```python
from build123d import *

# Parameters (mm, degrees)
BOSS_EXTRUDE1_DEPTH = 27
SHELL3_T            = -2
CUT_EXTRUDE1_DEPTH  = 2


with BuildPart() as part:
    # Sketch2 → Boss-Extrude1 (new body)
    with BuildSketch(Plane(origin=(0, 0, 0), x_dir=(1, 0, 0), z_dir=(0, 1, 0))):
        with BuildLine():
            Line((-18.993396104, 10.600093214), (-15.993396104, 10.600093214))
            ThreePointArc((-15.993396104, 10.600093214), (-12.085516583, 10.0001005), (-15.993393867, 9.400093214))
            Line((-15.993393867, 9.400093214), (-18.993393867, 9.400093214))
            ThreePointArc((-18.993393867, 9.400093214), (-19.274030957, 4.676202489), (-20, 0))
            Line((-20, 0), (0, 0))
            Line((0, 0), (0, 20))
            Line((0, 20), (-20, 20))
            ThreePointArc((-20, 20), (-19.274040883, 15.323890203), (-18.993396104, 10.600093214))
        make_face()
    extrude(amount=BOSS_EXTRUDE1_DEPTH)

    # Shell3
    shell3_openings = [part.faces().sort_by_distance(p)[0] for p in [
        (-19.274030957, 13.5, -4.676202489),
        (-17.493393867, 13.5, -9.400093214),
        (-12.085516583, 13.5, -10.0001005),
        (-17.493396104, 13.5, -10.600093214),
        (-19.274040883, 13.5, -15.323890203),
    ]]
    offset(amount=SHELL3_T, openings=shell3_openings, kind=Kind.INTERSECTION)

    # Sketch3 → Cut-Extrude1 (cut)
    with BuildSketch(Plane(origin=(0, 0, 0), x_dir=(0, 0, -1), z_dir=(1, 0, 0))):
        with BuildLine():
            ThreePointArc((12, 13.5), (10.89974713, 15.286184509), (8.809544899, 15.107114387))
            Line((8.809544899, 15.107114387), (11.190455101, 11.892885613))
            ThreePointArc((11.190455101, 11.892885613), (11.786184509, 12.60025287), (12, 13.5))
        make_face()
        with BuildLine():
            Line((11.190455101, 11.892885613), (8.809544899, 15.107114387))
            ThreePointArc((8.809544899, 15.107114387), (8.392885613, 12.309544899), (11.190455101, 11.892885613))
        make_face()
    extrude(amount=-CUT_EXTRUDE1_DEPTH, mode=Mode.SUBTRACT)


solid = part.part
```
Design review of the part built by this model. Coordinates are the model's own, in mm. A direction names the side the tool comes from. Coordinates: 2 decimals unless noted, no trailing zeros. Order: outer loops, then holes, each group sorted by start corner. A loop starts at its lowest first (then second) coordinate and runs counter-clockwise, first axis right, second up. Notation, with made-up numbers: (3.25, -20.75) - (25.25, -20.75) arc R21 cw to (25.25, -2.75) - close; hole circle Ø2 at (25, 68). An arc over 180 degrees is marked (long way). Answer in a Markdown table with one row per item.
(1) Clearance check with flat-ended pins moving along their axes: pin 1 (12 mm diameter, centred on y = 19, z = -13.5, fed in from -X); pin 2 (3.5 mm diameter, centred on x = -14.09, z = -10, fed in from -Y); pin 3 (4 mm diameter, centred on y = 13.5, z = -9.5, fed in from -X). State where each tip first meets the part, or that it passes through.
Checked values:
| item | result |
|---|---|
| pin 1 | x = -19.9 |
| pin 2 | through |
| pin 3 | x = -2 |
(2) Consider section B-B on x = -18. State the section outline as (y, z) points, plus the area to 3 significant figures.
Checked values:
| item | result |
|---|---|
| outline | (0, -20) - (27, -20) - (27, -10.6) - (25, -10.6) - (25, -18) - (2, -18) - (2, -10.6) - (0, -10.6) - close; (0, -9.4) - (2, -9.4) - (2, -2) - (25, -2) - (25, -9.4) - (27, -9.4) - (27, 0) - (0, 0) - close |
| area | 167 mm^2 |
(3) Wall thickness on line 1 along Y through (x, z) = (-6, -12); line 2 along Z through (x, y) = (-18.75, 8.5); line 3 along X through (y, z) = (21.75, -2.75): over which ranges is each line inside the solid? List them lowest first. Write a range as from..to.
Checked values:
| item | result |
|---|---|
| line 1 | 0..2, 25..27 |
| line 2 | -20..-18, -2..0 |
| line 3 | -2..0 |
(4) For faces 5 (the flat face through (-17, 1, -9.4)), 6 (the flat face through (-11, 13, -18)), 7 (the flat face through (-10, 27, -10)), list the 3-axis set-ups (+Z, -Z, +X, -X, +Y, -Y) from which the entire face can be reached by the end or side of a thin tool; tool diameter is ignored.
Checked values:
| item | result |
|---|---|
| face 5 | -X, +Y, -Y |
| face 6 | -X |
| face 7 | +Z, -Z, +X, -X, +Y |
(5) Consider section C-C on x = -9.25. State the section outline as (y, z) points.
Checked values:
| item | result |
|---|---|
| outline | (0, -20) - (27, -20) - (27, 0) - (0, 0) - close; hole (2, -18) - (25, -18) - (25, -2) - (2, -2) - close |
(6) The part is to be moulded in two halves that separate along Y. For faces 1 (the flat face through (-18, 26, -10.6)), 2 (the flat face through (-10, 0, -10)), 3 (the flat face through (-11, 25, -10)), 4 (the flat face through (-2, 16, -10)), say which applies: released by +Y, released by -Y, zero draft, split by the parting line, or undercut.
Checked values:
| item | result |
|---|---|
| face 1 | zero draft |
| face 2 | released by -Y |
| face 3 | undercut |
| face 4 | undercut |
(7) Consider section A-A on z = -10. State the section outline as (x, y) points.
Checked values:
| item | result |
|---|---|
| outline | (-12.09, 0) - (0, 0) - (0, 11.5) - (-2, 11.5) - (-2, 2) - (-12.09, 2) - close; (-12.09, 25) - (-2, 25) - (-2, 15.5) - (0, 15.5) - (0, 27) - (-12.09, 27) - close |
(8) Consider section D-D on y = 14.5. State the section outline as (x, z) points, plus the area to 3 significant figures.
Checked values:
| item | result |
|---|---|
| outline | (-20, -20) - (0, -20) - (0, -11.73) - (-2, -11.73) - (-2, -18) - (-19.63, -18) arc R50 cw to start; (-20, 0) arc R50 cw to (-19.63, -2) - (-2, -2) - (-2, -8.27) - (0, -8.27) - (0, 0) - close |
| area | 104 mm^2 |
